Check sheet for the modelled part. Datum: model origin and axes. Units: mm. A direction names the side the tool comes from. Round coordinates to 2 decimals unless told otherwise and drop trailing zeros. Write each loop counter-clockwise with the first axis right and the second up, starting at its lowest first coordinate (ties: lowest second). Pieces come first, ordered by that corner, then holes.
Item 1: Set-up check for faces 1 (the flat face through (-29.25, -1, 11)), 2 (the flat face through (19, 35, 8)), 3 (the cylindrical face through (29.511, 45.133, 10.846)): record each of +Z, -Z, +X, -X, +Y, -Y from which the full face is reachable in a straight line by a thin tool's end or side.
Item 2: Section check B-B, the plane x = -16.5. Record the cut outline in (y, z), plus the area to 4 significant figures.
Item 3: Section check A-A, the plane y = 42.5. Record the cut outline in (x, z).
Item 4: Section check C-C, the plane x = 16.5. Record the cut outline in (y, z), plus the area to 3 significant figures.
Item 5: Depth check by flat-ended pin: pin 1 (8 mm diameter, centred on x = 19.5, z = 6, fed in from -Y); pin 2 (2 mm diameter, centred on y = 39.5, z = 7.5, fed in from -X); pin 3 (4 mm diameter, centred on y = 31.5, z = 10, fed in from +X). Enter the tip coordinate at first touch or a pass-through.
Item 6: Release check for a two-part mould opening along Y. For faces 4 (the flat face through (2, -7, -5.5)), 5 (the flat face through (-22, -30, 7)) record: pulls with the +Y half, pulls with the -Y half, needs draft (parallel to the pull), parting line crosses it, or undercut.
Item 7: Section check D-D, the plane y = 32. Record the cut outline in (x, z), plus the area to 3 significant figures.
Item 8: Material ranges on line 1 along Y through (x, z) = (14.5, 7.5); line 2 along Y through (x, z) = (-26.5, 9.5); line 3 along X through (y, z) = (-34, 3), recorded low to high.
from build123d import *

# Parameters (mm, degrees)
F0_W      = 58.5
F0_H      = 91
F1_DEPTH  = 22
F2_T      = -1.5
F3_R      = 8.5
F4_DEPTH  = 25
F5_R      = 3
F6_R      = 2
F8_DEPTH  = 28
F9_W      = 2
F9_H      = 3
F9_R      = 4
F9_R_2    = 1.8
F10_DEPTH = 26
F11_R     = 4
F12_DEPTH = 22
F13_R     = 1.8
F14_DEPTH = 26
F16_SIZE  = 2


with BuildPart() as f1:
    # F0 (on Top) → F1 (new body)
    with BuildSketch(Plane.XY):
        Rectangle(F0_W, F0_H)
    extrude(amount=F1_DEPTH)

    # F2
    f2_openings = [f1.faces().sort_by_distance(p)[0] for p in [
        (0, 0, 0),
    ]]
    offset(amount=F2_T, openings=f2_openings)

    # F3 (on face) → F4 (cut)
    with BuildSketch(Plane.XY.offset(22)):
        with Locations((16.5, 17)):
            Circle(F3_R)
        with Locations((16.5, -17)):
            Circle(F3_R)
        with Locations((-16.5, -17)):
            Circle(F3_R)
    extrude(amount=-F4_DEPTH, mode=Mode.SUBTRACT)

    # F5
    f5_edges = [f1.edges().sort_by_distance(p)[0] for p in [
        (-29.25, 45.5, 11),
        (29.25, 45.5, 11),
        (-29.25, -45.5, 11),
        (29.25, -45.5, 11),
    ]]
    fillet(f5_edges, radius=F5_R)

    # F6
    f6_edges = [f1.edges().sort_by_distance(p)[0] for p in [
        (-27.75, 44, 10.25),
        (-27.75, -44, 10.25),
        (27.75, -44, 10.25),
        (27.75, 44, 10.25),
    ]]
    fillet(f6_edges, radius=F6_R)

    # F7 (on face) → F8 (join)
    with BuildSketch(Plane(origin=(0, 0, 20.5), x_dir=(1, 0, 0), z_dir=(0, 0, -1))):
        Polygon((12.5, 38), (20.5, 38), (20.5, 30), (22.5, 30), (22.5, 40), (12.5, 40), align=None)
        Polygon((20.5, -30), (20.5, -38), (12.5, -38), (12.5, -40), (22.5, -40), (22.5, -30), align=None)
        Polygon((-20.5, 30), (-20.5, 38), (-12.5, 38), (-12.5, 40), (-22.5, 40), (-22.5, 30), align=None)
        Polygon((-12.5, -40), (-12.5, -38), (-20.5, -38), (-20.5, -30), (-22.5, -30), (-22.5, -40), align=None)
    extrude(amount=F8_DEPTH)

    # F9 (on face) → F10 (join)
    with BuildSketch(Plane(origin=(0, 0, 20.5), x_dir=(1, 0, 0), z_dir=(0, 0, -1))):
        with Locations((19.5, 36.5)):
            Rectangle(F9_W, F9_H)
        with Locations((-19.5, 36.5)):
            Rectangle(F9_W, F9_H)
        with Locations((-19.5, -36.5)):
            Rectangle(F9_W, F9_H)
        with Locations((19.5, -36.5)):
            Rectangle(F9_W, F9_H)
        with Locations((0, 7.5)):
            Circle(F9_R)
        with Locations((0, 7.5)):
            Circle(F9_R_2, mode=Mode.SUBTRACT)
    extrude(amount=F10_DEPTH)

    # F11 (on face) → F12 (join)
    with BuildSketch(Plane.XY):
        with Locations((26.5, -42.5)):
            Circle(F11_R)
        with Locations((26.5, 42.5)):
            Circle(F11_R)
        with Locations((-26.5, 42.5)):
            Circle(F11_R)
        with Locations((-26.5, -42.5)):
            Circle(F11_R)
    extrude(amount=F12_DEPTH)

    # F13 (on Top) → F14 (cut)
    with BuildSketch(Plane.XY):
        with Locations((26.5, -42.5)):
            Circle(F13_R)
        with Locations((26.5, 42.5)):
            Circle(F13_R)
        with Locations((-26.5, -42.5)):
            Circle(F13_R)
        with Locations((-26.5, 42.5)):
            Circle(F13_R)
    extrude(amount=F14_DEPTH, mode=Mode.SUBTRACT)

    # F16
    f16_edges = [f1.edges().sort_by_distance(p)[0] for p in [
        (24.7, -42.5, 22),
        (24.7, 42.5, 22),
        (-28.3, 42.5, 22),
        (-28.3, -42.5, 22),
    ]]
    chamfer(f16_edges, length=F16_SIZE)


solid = f1.part
Values found:
1. face 1: +Z, -Z, -X
1. face 2: -Z
1. face 3: +Z, -Z
2. outline: (-45.5, 0) - (-44, 0) - (-44, 20.5) - (-40, 20.5) - (-40, -7.5) - (-38, -7.5) - (-38, 20.5) - (-25.5, 20.5) - (-25.5, 22) - (-45.5, 22) - close; (-8.5, 20.5) - (38, 20.5) - (38, -7.5) - (40, -7.5) - (40, 20.5) - (44, 20.5) - (44, 0) - (45.5, 0) - (45.5, 22) - (-8.5, 22) - close
2. area: 284.5 mm2
3. outline: (-30.5, 0) - (-28.3, 0) - (-28.3, 20) - (-30.3, 22) - (-30.5, 22) - close; (-24.7, 0) - (-22.5, 0) - (-22.5, 20.5) - (22.5, 20.5) - (22.5, 0) - (24.7, 0) - (24.7, 20) - (22.7, 22) - (-22.7, 22) - (-24.7, 20) - close; (28.3, 0) - (30.5, 0) - (30.5, 22) - (30.3, 22) - (28.3, 20) - close
4. outline: (-45.5, 0) - (-44, 0) - (-44, 20.5) - (-40, 20.5) - (-40, -7.5) - (-38, -7.5) - (-38, 20.5) - (-25.5, 20.5) - (-25.5, 22) - (-45.5, 22) - close; (-8.5, 20.5) - (8.5, 20.5) - (8.5, 22) - (-8.5, 22) - close; (25.5, 20.5) - (38, 20.5) - (38, -7.5) - (40, -7.5) - (40, 20.5) - (44, 20.5) - (44, 0) - (45.5, 0) - (45.5, 22) - (25.5, 22) - close
4. area: 259 mm2
5. pin 1: stops at y = -45.5
5. pin 2: stops at x = -29.96
5. pin 3: stops at x = 29.25
6. face 4: needs draft
6. face 5: undercut
7. outline: (-29.25, 0) - (-27.75, 0) - (-27.75, 20.5) - (-22.5, 20.5) - (-22.5, -7.5) - (-20.5, -7.5) - (-20.5, 20.5) - (20.5, 20.5) - (20.5, -7.5) - (22.5, -7.5) - (22.5, 20.5) - (27.75, 20.5) - (27.75, 0) - (29.25, 0) - (29.25, 22) - (-29.25, 22) - close
7. area: 261 mm2
8. line 1: y = -45.5 to -44, -40 to -38, 38 to 40, 44 to 45.5
8. line 2: y = -46.5 to -44.3, -40.7 to -38.5, 38.5 to 40.7, 44.3 to 46.5
8. line 3: x = -29.25 to -27.75, -22.5 to -20.5, 20.5 to 22.5, 27.75 to 29.25
